Input: part model. Units: mm. Frame: model coordinates. A direction names the side the tool comes from. Round coordinates to 2 decimals unless told otherwise and drop trailing zeros. Order: outer loops, then holes, each group sorted by start corner. A loop starts at its lowest first (then second) coordinate and runs counter-clockwise, first axis right, second up. Notation, with made-up numbers: M 86.5,74 L 111.5,74 A17 ccw 111.5,101 Z; hole C 20,47.5 d3. An arc over 180 degrees is marked long. One line per question, with ' | ' between items.
```python
from build123d import *

# Parameters (mm, degrees)
SKETCH_1_R          = 6
EXTRUDE_1_DEPTH     = 116
CUT_EXTRUDE_START   = -13.2
SKETCH_2_OUTSIDE_W  = 37.446
SKETCH_2_OUTSIDE_H  = 37.446
SKETCH_2_OUTSIDE_R  = 5.5
CUT_EXTRUDE_1_DEPTH = 1.2
CUT_EXTRUDE_START_2 = -40
SKETCH_3_OUTSIDE_W  = 37.446
SKETCH_3_OUTSIDE_H  = 37.446
SKETCH_3_OUTSIDE_R  = 5.5
CUT_EXTRUDE_2_DEPTH = 1.2
CUT_EXTRUDE_3_DEPTH = 13.2
CHAMFER_1_SIZE      = 1
SKETCH_5_OUTSIDE_W  = 37.446
SKETCH_5_OUTSIDE_H  = 37.446
CUT_EXTRUDE_4_DEPTH = 45


with BuildPart() as part:
    # 草图1 → 凸台-拉伸1 (new body)
    with BuildSketch(Plane.XY):
        with Locations(Location((0, 0, 0), (0, 0, 180))):
            Circle(SKETCH_1_R)
    extrude(amount=EXTRUDE_1_DEPTH)

    # 草图2 outside → 切除-拉伸1 (cut)
    with BuildSketch(Plane.XY.offset(116).offset(CUT_EXTRUDE_START)):
        Rectangle(SKETCH_2_OUTSIDE_W, SKETCH_2_OUTSIDE_H)
        Circle(SKETCH_2_OUTSIDE_R, mode=Mode.SUBTRACT)
    extrude(amount=CUT_EXTRUDE_1_DEPTH, mode=Mode.SUBTRACT)

    # 草图3 outside → 切除-拉伸2 (cut)
    with BuildSketch(Plane.XY.offset(102.8).offset(CUT_EXTRUDE_START_2)):
        Rectangle(SKETCH_3_OUTSIDE_W, SKETCH_3_OUTSIDE_H)
        Circle(SKETCH_3_OUTSIDE_R, mode=Mode.SUBTRACT)
    extrude(amount=-CUT_EXTRUDE_2_DEPTH, mode=Mode.SUBTRACT)

    # 草图4 → 切除-拉伸3 (cut)
    with BuildSketch(Plane.XY.offset(116).offset(CUT_EXTRUDE_START)):
        with BuildLine():
            Line((-1, 4.898979486), (-1, 5.916079783))
            ThreePointArc((-1, 5.916079783), (-2.296100594, 5.543277195), (-3.476193351, 4.890406914))
            Line((-3.476193351, 4.890406914), (-2.756994834, 4.171208396))
            ThreePointArc((-2.756994834, 4.171208396), (-1.913417162, 4.619397663), (-1, 4.898979486))
        make_face()
        with BuildLine():
            Line((1, 4.898979486), (1, 5.916079783))
            ThreePointArc((1, 5.916079783), (2.296100594, 5.543277195), (3.476193351, 4.890406914))
            Line((3.476193351, 4.890406914), (2.756994834, 4.171208396))
            ThreePointArc((2.756994834, 4.171208396), (1.913417162, 4.619397663), (1, 4.898979486))
        make_face()
        with BuildLine():
            Line((4.171208396, 2.756994834), (4.890406914, 3.476193351))
            ThreePointArc((4.890406914, 3.476193351), (5.543277195, 2.296100594), (5.916079783, 1))
            Line((5.916079783, 1), (4.898979486, 1))
            ThreePointArc((4.898979486, 1), (4.619397663, 1.913417162), (4.171208396, 2.756994834))
        make_face()
        with BuildLine():
            Line((4.898979486, -1), (5.916079783, -1))
            ThreePointArc((5.916079783, -1), (5.543277195, -2.296100594), (4.890406914, -3.476193351))
            Line((4.890406914, -3.476193351), (4.171208396, -2.756994834))
            ThreePointArc((4.171208396, -2.756994834), (4.619397663, -1.913417162), (4.898979486, -1))
        make_face()
        with BuildLine():
            Line((2.756994834, -4.171208396), (3.476193351, -4.890406914))
            ThreePointArc((3.476193351, -4.890406914), (2.296100594, -5.543277195), (1, -5.916079783))
            Line((1, -5.916079783), (1, -4.898979486))
            ThreePointArc((1, -4.898979486), (1.913417162, -4.619397663), (2.756994834, -4.171208396))
        make_face()
        with BuildLine():
            Line((-1, -4.898979486), (-1, -5.916079783))
            ThreePointArc((-1, -5.916079783), (-2.296100594, -5.543277195), (-3.476193351, -4.890406914))
            Line((-3.476193351, -4.890406914), (-2.756994834, -4.171208396))
            ThreePointArc((-2.756994834, -4.171208396), (-1.913417162, -4.619397663), (-1, -4.898979486))
        make_face()
        with BuildLine():
            Line((-4.171208396, -2.756994834), (-4.890406914, -3.476193351))
            ThreePointArc((-4.890406914, -3.476193351), (-5.543277195, -2.296100594), (-5.916079783, -1))
            Line((-5.916079783, -1), (-4.898979486, -1))
            ThreePointArc((-4.898979486, -1), (-4.619397663, -1.913417162), (-4.171208396, -2.756994834))
        make_face()
        with BuildLine():
            Line((-4.898979486, 1), (-5.916079783, 1))
            ThreePointArc((-5.916079783, 1), (-5.543277195, 2.296100594), (-4.890406914, 3.476193351))
            Line((-4.890406914, 3.476193351), (-4.171208396, 2.756994834))
            ThreePointArc((-4.171208396, 2.756994834), (-4.619397663, 1.913417162), (-4.898979486, 1))
        make_face()
    extrude(amount=CUT_EXTRUDE_3_DEPTH, mode=Mode.SUBTRACT)

    # 倒角1
    chamfer_1_edges = [part.edges().sort_by_distance(p)[0] for p in [
        (6, 0, 0),
    ]]
    chamfer(chamfer_1_edges, length=CHAMFER_1_SIZE)

    # 草图5 outside → 切除-拉伸4 (cut)
    with BuildSketch(Plane(origin=(0, 0, 0), x_dir=(-1, 0, 0), z_dir=(0, 0, -1))):
        Rectangle(SKETCH_5_OUTSIDE_W, SKETCH_5_OUTSIDE_H)
        Polygon((0, -6.363961031), (6.363961031, 0), (0, 6.363961031), (-6.363961031, 0), align=None, mode=Mode.SUBTRACT)
    extrude(amount=-CUT_EXTRUDE_4_DEPTH, mode=Mode.SUBTRACT)


solid = part.part
```
Item 1: First-contact query: pin 1 (0.7 mm diameter, centred on x = 0.5, y = 5.5, fed in from -Z); pin 2 (1.5 mm diameter, centred on y = 3, z = 76.5, fed in from -X); pin 3 (2 mm diameter, centred on y = 3, z = 19.5, fed in from -X). Flat tips, straight axial feed; report the tip coordinate or a pass-through.
Report:
pin 1: z = 0.17 | pin 2: x = -5.56 | pin 3: x = -4.36
Item 2: Mould query, pull axis Z, two halves, no side actions, for faces 1 (the flat face through (3.143, 3.221, 22.185)), 2 (the flat face through (-4, 4, 45)), 3 (the flat face through (2, -5, 102.8)). Classes: +Z half, -Z half, draft (parallel to the pull), parting line (faces both ways), or undercut.
Report:
face 1: draft | face 2: -Z half | face 3: undercut
Item 3: Section query A-A, the plane z = 28. Return loops of the section in (x, y).
Report:
outline: M -5.99,-0.38 L -0.38,-5.99 A6 ccw 0.38,-5.99 L 5.99,-0.38 A6 ccw 5.99,0.38 L 0.38,5.99 A6 ccw -0.38,5.99 L -5.99,0.38 A6 ccw Z
Item 4: Line query: line 1 along Y through (x, z) = (-0.25, 41); line 2 along Y through (x, z) = (-3.25, 44.5); line 3 along X through (y, z) = (5.25, 104). Output: solid intervals per line, ascending. Write a range as from..to.
Report:
line 1: -5.99..5.99 | line 2: -3.11..3.11 | line 3: -1..1
Item 5: Access query for faces 4 (the flat face through (3, -5, 61.6)), 5 (the flat face through (3.221, -3.143, 22.185)), 6 (the flat face through (-3.221, 3.143, 22.185)). Directions: +Z, -Z, +X, -X, +Y, -Y. A direction counts if a zero-diameter tool reaches every point of the face in a straight line with its end or side. Return the directions, or none.
Report:
face 4: none | face 5: -Z, +X, -Y | face 6: -Z, -X, +Y
Item 6: Section query B-B, the plane z = 91.5. Return loops of the section in (x, y).
Report:
outline: C 0,0 d12
